Could you check a few things on this model? Use its own coordinates, in mm. A direction names the side the tool comes from. Give positions to 0.01 mm unless a question says otherwise; leave off trailing zeros. Write each loop counter-clockwise with the first axis right and the second up, starting at its lowest first coordinate (ties: lowest second). Pieces come first, ordered by that corner, then holes. Notation, with made-up numbers: M 3.5,-28 L 49.5,-28 A13 cw 49.5,-11 Z; hole C -32,-27.5 d7. An arc over 180 degrees is marked long. One line per item, written item: value.
```python
from build123d import *

# Parameters (mm, degrees)
SKETCH1_W           = 70
SKETCH1_H           = 50
BOSS_EXTRUDE1_DEPTH = 2
SKETCH2_W           = 2
SKETCH2_H           = 50
BOSS_EXTRUDE2_DEPTH = 37
SKETCH3_W           = 12
SKETCH3_H           = 50
BOSS_EXTRUDE3_DEPTH = 2
SKETCH4_R           = 5
SKETCH4_R_2         = 2
CUT_EXTRUDE1_DEPTH  = 2
SKETCH5_R           = 7.75
SKETCH5_R_2         = 1.5
CUT_EXTRUDE2_DEPTH  = 2
SKETCH6_R           = 1.5
CUT_EXTRUDE3_DEPTH  = 2


with BuildPart() as part:
    # Sketch1 → Boss-Extrude1 (new body)
    with BuildSketch(Plane.XY):
        Rectangle(SKETCH1_W, SKETCH1_H)
    extrude(amount=BOSS_EXTRUDE1_DEPTH)

    # Sketch2 → Boss-Extrude2 (add)
    with BuildSketch(Plane.XY.offset(2)):
        with Locations((34, 0)):
            Rectangle(SKETCH2_W, SKETCH2_H)
        with Locations((-34, 0)):
            Rectangle(SKETCH2_W, SKETCH2_H)
    extrude(amount=BOSS_EXTRUDE2_DEPTH)

    # Sketch3 → Boss-Extrude3 (add)
    with BuildSketch(Plane.XY.offset(39)):
        with Locations((39, 0)):
            Rectangle(SKETCH3_W, SKETCH3_H)
        with Locations((-39, 0)):
            Rectangle(SKETCH3_W, SKETCH3_H)
    extrude(amount=BOSS_EXTRUDE3_DEPTH)

    # Sketch4 → Cut-Extrude1 (cut)
    with BuildSketch(Plane(origin=(35, 0, 0), x_dir=(0, 0, -1), z_dir=(1, 0, 0))):
        with Locations(Location((-29, 0, 0), (0, 0, 90))):
            Circle(SKETCH4_R)
        with Locations(Location((-21, 17.5, 0), (0, 0, 90))):
            Circle(SKETCH4_R_2)
        with Locations(Location((-21, -17.5, 0), (0, 0, 90))):
            Circle(SKETCH4_R_2)
    extrude(amount=-CUT_EXTRUDE1_DEPTH, mode=Mode.SUBTRACT)

    # Sketch5 → Cut-Extrude2 (cut)
    with BuildSketch(Plane.ZY.offset(35)):
        with Locations(Location((29, 0, 0), (0, 0, 270))):
            Circle(SKETCH5_R)
        with Locations(Location((29, 15, 0), (0, 0, 270))):
            Circle(SKETCH5_R_2)
        with Locations(Location((29, -15, 0), (0, 0, 270))):
            Circle(SKETCH5_R_2)
    extrude(amount=-CUT_EXTRUDE2_DEPTH, mode=Mode.SUBTRACT)

    # Sketch6 → Cut-Extrude3 (cut)
    with BuildSketch(Plane(origin=(0, 0, 39), x_dir=(-1, 0, 0), z_dir=(0, 0, -1))):
        with Locations((-40, 15)):
            Circle(SKETCH6_R)
        with Locations(Location((-40, -15, 0), (0, 0, 180))):
            Circle(SKETCH6_R)
        with Locations((40, -15)):
            Circle(SKETCH6_R)
        with Locations(Location((40, 15, 0), (0, 0, 180))):
            Circle(SKETCH6_R)
    extrude(amount=-CUT_EXTRUDE3_DEPTH, mode=Mode.SUBTRACT)


solid = part.part
```
1) If we section it at D-D, the plane y = 1: Write out the boundary of the cut face in (x, z).
Outcome:
outline: M -45,39 L -35,39 L -35,36.69 L -33,36.69 L -33,41 L -45,41 Z; M -35,0 L 35,0 L 35,24.1 L 33,24.1 L 33,2 L -33,2 L -33,21.31 L -35,21.31 Z; M 33,33.9 L 35,33.9 L 35,39 L 45,39 L 45,41 L 33,41 Z
2) If we section it at A-A, the plane x = 40: Write out the boundary of the cut face in (y, z).
Outcome:
outline: M -25,39 L -16.5,39 L -16.5,41 L -25,41 Z; M -13.5,39 L 13.5,39 L 13.5,41 L -13.5,41 Z; M 16.5,39 L 25,39 L 25,41 L 16.5,41 Z
3) We'd pull the mould along X, two halves only. Please class faces 5 (the face through (-45, 0, 40)), 6 (the face through (45, 0, 40)), 7 (the face through (-34.014, 1.009, 36.684)), 8 (the face through (-41.5, 14.93, 39.99)): pulls with the +X half, pulls with the -X half, needs draft (parallel to the pull), parting line crosses it, or undercut.
Outcome:
face 5: pulls with the -X half
face 6: pulls with the +X half
face 7: needs draft
face 8: undercut
4) On a 3-axis mill with a long thin cutter (end or side, diameter ignored), from which of +Z, -Z, +X, -X, +Y, -Y can I reach the whole of each face in a straight line? I mean faces 1 (the face through (-34.01, 16.11, 30.01)), 2 (the face through (35, 0, 19)), 3 (the face through (33, 0, 21)), 4 (the face through (-40, 0, 39)). Say none if no direction works.
Outcome:
face 1: -X
face 2: -Z, +X, +Y, -Y
face 3: +Z, +Y, -Y
face 4: -Z, -X, +Y, -Y
5) Please list where these lines run through material, in increasing order: L1, parallel to Y at x = 40, z = 40; L2, parallel to X at y = 0, z = 19.5; L3, parallel to Z at x = -34.25, y = -15. Write a range as from..to.
Outcome:
L1: y = -25..-16.5, -13.5..13.5, 16.5..25
L2: x = -35..-33, 33..35
L3: z = 0..27.5, 30.5..41
6) I'm going to push flat-ended pins straight in: pin 1 (4 mm diameter, centred on x = 40, y = 15, fed in from -Z); pin 2 (1 mm diameter, centred on y = 9, z = 27, fed in from -X); pin 3 (19.5 mm diameter, centred on y = -7, z = 29, fed in from +X); pin 4 (2.5 mm diameter, centred on x = -40, y = -15, fed in from +Z). Where does each tip first touch, or does it pass through?
Outcome:
pin 1: stops at z = 39
pin 2: stops at x = -35
pin 3: stops at x = 35
pin 4: passes through
7) If we section it at B-B, the plane z = 3.5: Write out the boundary of the cut face in (x, y).
Outcome:
outline: M -35,-25 L -33,-25 L -33,25 L -35,25 Z; M 33,-25 L 35,-25 L 35,25 L 33,25 Z
8) If we section it at C-C, the plane y = 17.5: Write out the boundary of the cut face in (x, z).
Outcome:
outline: M -45,39 L -35,39 L -35,0 L 35,0 L 35,19 L 33,19 L 33,2 L -33,2 L -33,41 L -45,41 Z; M 33,23 L 35,23 L 35,39 L 45,39 L 45,41 L 33,41 Z
